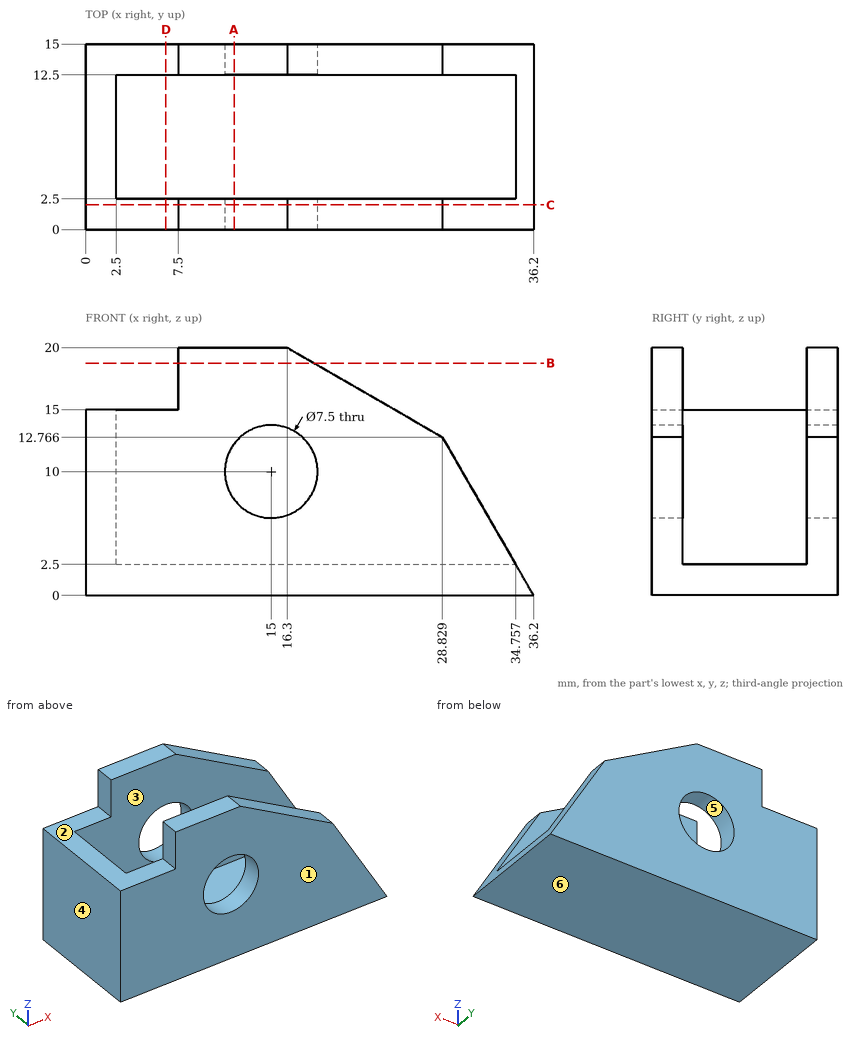
Here's the drawing with two shaded views (mm, measured from the low corner). I have some questions. A direction names the side the tool comes from. Give positions to 0.01 mm unless a question says otherwise; leave off trailing zeros. Write each loop counter-clockwise with the first axis right and the second up, starting at its lowest first coordinate (ties: lowest second). Pieces come first, ordered by that corner, then holes. Notation, with made-up numbers: (-19.5, 67.5) - (3.5, 67.5) arc R24 cw to (3.5, 87.5) - close; hole circle Ø8 at (29, 87). An arc over 180 degrees is marked (long way). One line per item, written item: value. Start each with the question number.
Item 1: Imagine slicing it at C-C, the plane y = 2. List the corners of the cut face in (x, z) for me, and give its area (3 significant figures).
Item 2: Which directions (+Z, -Z, +X, -X, +Y, -Y) give clear straight access to the entire face, cutting with the end or side of a thin tool? Please do the marked faces 1, 2 and 3.
Item 3: Imagine slicing it at B-B, the plane z = 18.75. List the corners of the cut face in (x, y) for me (1 decimal).
Item 4: Imagine slicing it at D-D, the plane x = 6.5. List the corners of the cut face in (y, z) for me, and give its area (3 significant figures).
Item 5: Imagine slicing it at A-A, the plane x = 12. List the corners of the cut face in (y, z) for me.
Item 6: I'm going to push flat-ended pins straight in: pin 1 (2 mm diameter, centred on y = 14, z = 17.5, fed in from -X); pin 2 (5 mm diameter, centred on y = 6, z = 8.5, fed in from +X); pin 3 (2 mm diameter, centred on x = 5, y = 10, fed in from +Z); pin 4 (7 mm diameter, centred on x = 15, z = 10, fed in from +Y). Where does each tip first touch, or does it pass through?
Item 7: Please list where these lines run through material, in increasing order: line 1 (Y direction, x = 25, z = 6.75); line 2 (Z direction, x = 15, y = 1.9); line 3 (Z direction, x = 7.5, y = 10.5). Write a range as from..to.
Item 8: If we mould it in two halves opening along Z, with no side actions, what happens to the marked faces 4, 5 and 6? For each: +Z half, -Z half, draft (parallel to the pull), parting line (faces both ways), or undercut.
Geometry says:
1. outline: (0, 0) - (36.2, 0) - (28.83, 12.77) - (16.3, 20) - (7.5, 20) - (7.5, 15) - (0, 15) - close; hole circle Ø7.5 at (15, 10)
1. area: 497 mm^2
2. face 1: +Z, -Z, +X, -X, -Y
2. face 2: +Z, -X, +Y, -Y
2. face 3: +Z, +X
3. outline: (7.5, 0) - (18.5, 0) - (18.5, 2.5) - (7.5, 2.5) - close; (7.5, 12.5) - (18.5, 12.5) - (18.5, 15) - (7.5, 15) - close
4. outline: (0, 0) - (15, 0) - (15, 15) - (12.5, 15) - (12.5, 2.5) - (2.5, 2.5) - (2.5, 15) - (0, 15) - close
4. area: 100 mm^2
5. outline: (0, 0) - (15, 0) - (15, 7.75) - (12.5, 7.75) - (12.5, 2.5) - (2.5, 2.5) - (2.5, 7.75) - (0, 7.75) - close; (0, 12.25) - (2.5, 12.25) - (2.5, 20) - (0, 20) - close; (12.5, 12.25) - (15, 12.25) - (15, 20) - (12.5, 20) - close
6. pin 1: x = 7.5
6. pin 2: x = 2.5
6. pin 3: z = 2.5
6. pin 4: through
7. line 1: 0..2.5, 12.5..15
7. line 2: 0..6.25, 13.75..20
7. line 3: 0..2.5
8. face 4: draft
8. face 5: undercut
8. face 6: -Z half
